Could you check a few things on this drawing? It's one solid part, dimensions in mm from its lowest x, y, z. A direction names the side the tool comes from. Give positions to 0.01 mm unless a question says otherwise; leave off trailing zeros. Loops run counter-clockwise (first coordinate to the right, second up) from the corner with the lowest first, then second, coordinate; pieces in that order, holes last. Notation, with made-up numbers: M 57.5,58 L 104.5,58 A29 ccw 104.5,93 Z; hole C 69.25,-16.5 d9. An arc over 180 degrees is marked long. Return JSON: item names as keys, results as strings. Group by question number.
1. If we section it at A-A (x = 41.5): Write out the boundary of the cut face in (y, z), plus the area to 3 significant figures.
2. For the marked faces 1, 2, 3, 4 and 5, which set-ups out of +Z, -Z, +X, -X, +Y, -Y let a thin tool reach every point of the face, with its end or its side?
3. If we section it at B-B (y = 25.4): Write out the boundary of the cut face in (x, z), plus the area to 3 significant figures.
4. If we section it at C-C (z = 36): Write out the boundary of the cut face in (x, y), plus the area to 3 significant figures.
5. If we mould it in two halves opening along Z, with no side actions, what happens to the marked faces 6, 7 and 8? For each: +Z half, -Z half, draft (parallel to the pull), parting line (faces both ways), or undercut.
6. Please list where these lines run through material, in increasing order: line 1 (Y direction, x = 33, z = 12.7); line 2 (Z direction, x = 44, y = 25); line 3 (Z direction, x = 36, y = 25).
7. If we section it at D-D (z = 15): Write out the boundary of the cut face in (x, y), plus the area to 3 significant figures.
8. For pin 1 (15 mm diameter, centred on x = 64.5, y = 42.5, fed in from +Z); pin 2 (6.5 mm diameter, centred on y = 8, z = 44.5, fed in from +X); pin 3 (4 mm diameter, centred on x = 36, y = 47, fed in from +Z); pin 4 (11.5 mm diameter, centred on y = 25.4, z = 12.7, fed in from +X), each with a flat end and sliding along its axis, tell me the tip position at first contact or that it passes through.
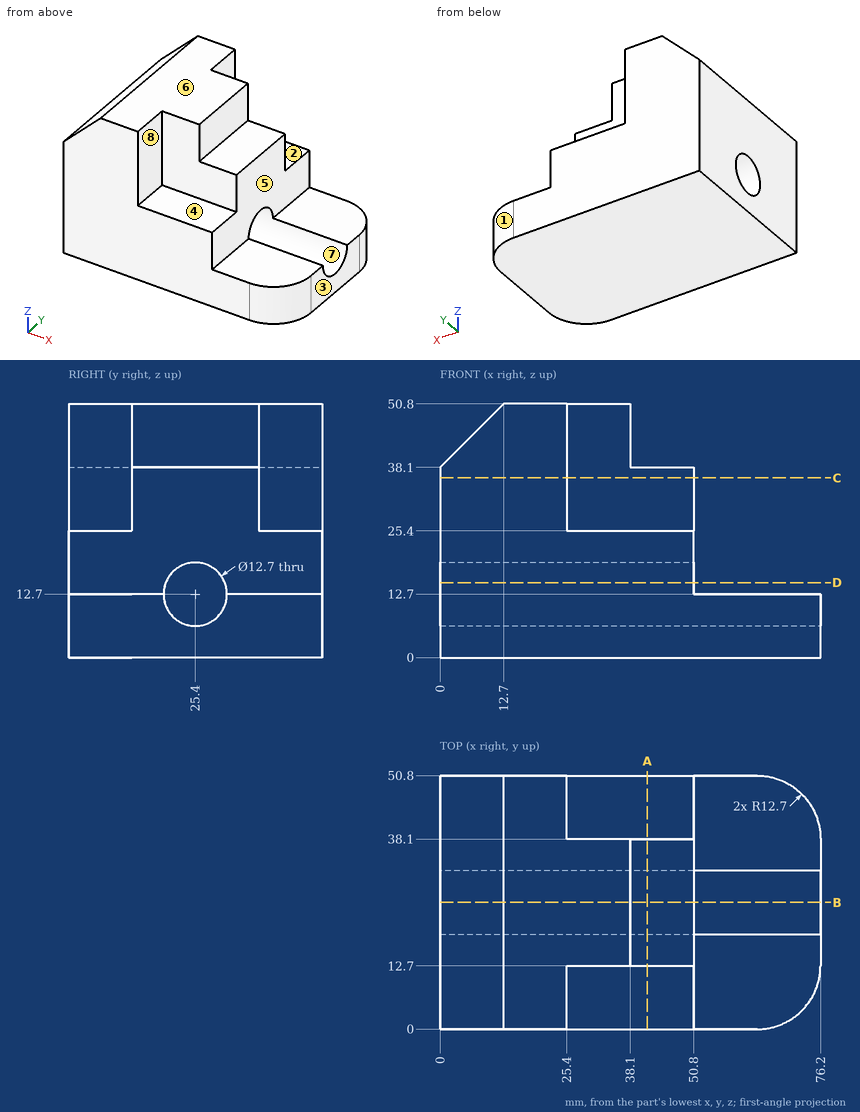
Answer:
{
 "1": {"outline": "M 0,0 L 50.8,0 L 50.8,25.4 L 38.1,25.4 L 38.1,38.1 L 12.7,38.1 L 12.7,25.4 L 0,25.4 Z; hole C 25.4,12.7 d12.7", "area": "1,490 mm²"},
 "2": {"face 1": "+Z, -Z, +X, +Y", "face 2": "+Z, +X, +Y", "face 3": "+Z, -Z, +X, +Y, -Y", "face 4": "+Z, +X, -Y", "face 5": "+Z, +X, +Y, -Y"},
 "3": {"outline": "M 0,0 L 76.2,0 L 76.2,6.35 L 0,6.35 Z; M 0,19.05 L 50.8,19.05 L 50.8,38.1 L 38.1,38.1 L 38.1,50.8 L 12.7,50.8 L 0,38.1 Z", "area": "1,850 mm²"},
 "4": {"outline": "M 0,0 L 25.4,0 L 25.4,12.7 L 50.8,12.7 L 50.8,38.1 L 25.4,38.1 L 25.4,50.8 L 0,50.8 Z", "area": "1,940 mm²"},
 "5": {"face 6": "+Z half", "face 7": "undercut", "face 8": "draft"},
 "6": {"line 1": "y = 0 to 19.05, 31.75 to 50.8", "line 2": "z = 0 to 6.36, 19.04 to 38.1", "line 3": "z = 0 to 6.36, 19.04 to 50.8"},
 "7": {"outline": "M 0,0 L 50.8,0 L 50.8,19.48 L 0,19.48 Z; M 0,31.32 L 50.8,31.32 L 50.8,50.8 L 0,50.8 Z", "area": "1,980 mm²"},
 "8": {"pin 1": "stops at z = 12.7", "pin 2": "stops at x = 25.4", "pin 3": "stops at z = 25.4", "pin 4": "passes through"}
}
